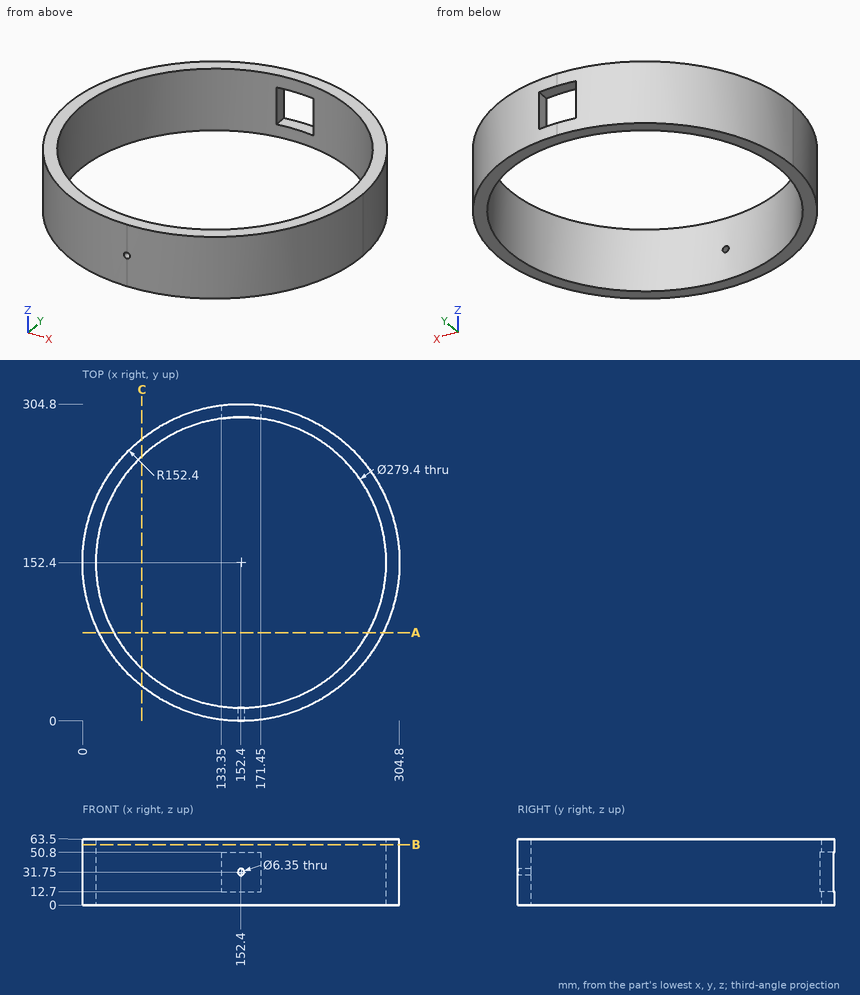
Here's the drawing with two shaded views (mm, measured from the low corner). I have some questions. Give positions to 0.01 mm unless a question says otherwise; leave off trailing zeros. Write each loop counter-clockwise with the first axis right and the second up, starting at its lowest first coordinate (ties: lowest second). Pieces come first, ordered by that corner, then holes. Notation, with made-up numbers: (6.5, 54) - (13.5, 54) arc R8 cw to (13.5, 68) - close; hole circle Ø6 at (17, 65). An arc over 180 degrees is marked (long way). One line per item, written item: value. Start each with the question number.
Item 1: Please list where these lines run through material, in increasing order: line 1 (Y direction, x = 148.5, z = 10.5); line 2 (X direction, y = 152, z = 49); line 3 (X direction, y = 171, z = 61.5). Write a range as from..to.
Item 2: Imagine slicing it at C-C, the plane x = 57. List the corners of the cut face in (y, z) for me, and give its area (3 significant figures).
Item 3: I'm going to push flat-ended pins straight in: pin 1 (3 mm diameter, centred on x = 55, z = 46.5, fed in from -Y); pin 2 (1 mm diameter, centred on y = 262.5, z = 31.5, fed in from -X); pin 3 (12 mm diameter, centred on x = 235, z = 23, fed in from +Y). Where does each tip first touch, or does it pass through?
Item 4: Imagine slicing it at B-B, the plane z = 58. List the corners of the cut face in (x, y) for me, and give its area (3 significant figures).
Item 5: Imagine slicing it at A-A, the plane y = 85. List the corners of the cut face in (x, z) for me.
Geometry says:
1. line 1: 0.05..12.75, 292.05..304.75
1. line 2: 0..12.7, 292.1..304.8
1. line 3: 1.14..13.94, 290.86..303.66
2. outline: (33.55, 0) - (50.35, 0) - (50.35, 63.5) - (33.55, 63.5) - close; (254.45, 0) - (271.25, 0) - (271.25, 63.5) - (254.45, 63.5) - close
2. area: 2,130 mm^2
3. pin 1: y = 33.96
3. pin 2: x = 46.51
3. pin 3: y = 284.15
4. outline: circle Ø304.8 at (152.4, 152.4); hole circle Ø279.4 at (152.4, 152.4)
4. area: 11,700 mm^2
5. outline: (15.71, 0) - (30.03, 0) - (30.03, 63.5) - (15.71, 63.5) - close; (274.77, 0) - (289.09, 0) - (289.09, 63.5) - (274.77, 63.5) - close
